Part model, mm, in its own coordinate system. A direction names the side the tool comes from. Round coordinates to 2 decimals unless told otherwise and drop trailing zeros. Write each loop counter-clockwise with the first axis right and the second up, starting at its lowest first coordinate (ties: lowest second). Pieces come first, ordered by that corner, then holes. Notation, with made-up numbers: (73, -0.75) -> (131, -0.75) arc R32 cw to (131, 34.25) -> close; hole circle Ø3 at (-16.75, -36). An arc over 180 degrees is marked (long way). Return JSON: item names as keys, results as strings. Group by question number.
(1) Tool access for faces 4 (the flat face through (-26, 33, -3)), 5 (the flat face through (-49, 32, 198.75)), 6 (the flat face through (2, -19, -198.75)): list every direction of +Z, -Z, +X, -X, +Y, -Y with a clear straight run to the whole face (end or side of a thin tool).
(2) Saw through at C-C (y = 47.5). List the corners of the cut face in (x, z).
(3) Saw through at B-B (x = -12.5). List the corners of the cut face in (y, z).
(4) Mould opens along Z. For faces 1 (the flat face through (2, 0, -3)), 2 (the flat face through (-48, 33, -202.75)), 3 (the cylindrical face through (-43.53, 21.38, 200.78)) say: +Z half, -Z half, draft (parallel to the pull), parting line (faces both ways), or undercut.
(5) Saw through at A-A (z = 122.75). List the corners of the cut face in (x, y), plus the area to 3 significant figures.
(6) Saw through at D-D (z = 3.5). List the corners of the cut face in (x, y).
(7) Drill centre lines: L1, parallel to Z at x = -48, y = 42; L2, parallel to Y at x = 4, z = -93.5; L3, parallel to Y at x = -12, z = 200. Where is each one in solid material? Low to high. Write a range as from..to.
(8) Drop flat-ended pins along their axis: pin 1 Ø1 at (y, z) = (19, -57) entering from +X; pin 2 Ø7.5 at (y, z) = (35, -122.75) entering from -X; pin 3 Ø1.5 at (y, z) = (-9.5, -199) entering from -X; pin 4 Ø3 at (y, z) = (38.5, 108.5) entering from -X. Give the stop position or say it passes through.
from build123d import *

# Parameters (mm, degrees)
SKETCH1_W                      = 60
SKETCH1_H                      = 405.5
BASE_FLANGE1_DEPTH             = 4
EDGE_FLANGE1_STRIP_W           = 18
EDGE_FLANGE1_STRIP_H           = 4
EDGE_FLANGE1_STRIP_CUT_DEPTH   = 405.5
EDGE_FLANGE1_DEPTH             = 405.5
EDGE_FLANGE2_STRIP_W           = 18
EDGE_FLANGE2_STRIP_H           = 4
EDGE_FLANGE2_STRIP_CUT_DEPTH   = 55
EDGE_FLANGE2_STRIP_2_W         = 18
EDGE_FLANGE2_STRIP_2_H         = 4
EDGE_FLANGE2_STRIP_CUT_2_DEPTH = 55
EDGE_FLANGE2_STRIP_3_W         = 18
EDGE_FLANGE2_STRIP_3_H         = 4
EDGE_FLANGE2_STRIP_CUT_3_DEPTH = 55
EDGE_FLANGE2_STRIP_4_W         = 18
EDGE_FLANGE2_STRIP_4_H         = 4
EDGE_FLANGE2_STRIP_CUT_4_DEPTH = 55
EDGE_FLANGE2_DEPTH             = 55
EDGE_FLANGE2_BEND_DEPTH        = 55
EDGE_FLANGE2_BEND_2_DEPTH      = 55
EDGE_FLANGE2_BEND_3_DEPTH      = 55
SKETCH18_R                     = 4.6
EXTRUDE1_DEPTH                 = 416.194231655
SKETCH19_R                     = 4.6
EXTRUDE2_DEPTH                 = 4
SKETCH20_R                     = 4.6
EXTRUDE3_DEPTH                 = 4


# Sheet-metal steps are written as plain solids
with BuildPart() as part:
    # Sketch1 → Base-Flange1 (new body)
    with BuildSketch(Plane(origin=(0, 0, 0), x_dir=(1, 0, 0), z_dir=(0, 1, 0))):
        Rectangle(SKETCH1_W, SKETCH1_H)
    extrude(amount=BASE_FLANGE1_DEPTH)

    # Edge-Flange1 strip (across the edge) → Edge-Flange1 strip cut (cut)
    with BuildSketch(Plane(origin=(-30, 4, -202.75), x_dir=(1, 0, 0), z_dir=(0, 0, 1))):
        with Locations((-4, -2)):
            Rectangle(EDGE_FLANGE1_STRIP_W, EDGE_FLANGE1_STRIP_H)
    extrude(amount=EDGE_FLANGE1_STRIP_CUT_DEPTH, mode=Mode.SUBTRACT)

    # Edge-Flange1 section (across the edge) → Edge-Flange1 (add)
    with BuildSketch(Plane(origin=(-30, 4, -202.75), x_dir=(1, 0, 0), z_dir=(0, 0, 1))):
        with BuildLine():
            Line((0, 1), (0, 56))
            Line((0, 56), (4, 56))
            Line((4, 56), (4, 1))
            ThreePointArc((4, 1), (4.292893219, 0.292893219), (5, 0))
            Line((5, 0), (5, -4))
            ThreePointArc((5, -4), (1.464466094, -2.535533906), (0, 1))
        make_face()
    extrude(amount=EDGE_FLANGE1_DEPTH)

    # Edge-Flange2 strip (across the edge) → Edge-Flange2 strip cut (cut)
    with BuildSketch(Plane(origin=(-30, 5, 202.75), x_dir=(0, 0, -1), z_dir=(0, 1, 0))):
        with Locations((-4, -2)):
            Rectangle(EDGE_FLANGE2_STRIP_W, EDGE_FLANGE2_STRIP_H)
    extrude(amount=EDGE_FLANGE2_STRIP_CUT_DEPTH, mode=Mode.SUBTRACT)

    # Edge-Flange2 strip 2 (across the edge) → Edge-Flange2 strip cut 2 (cut)
    with BuildSketch(Plane(origin=(30, 0, 202.75), x_dir=(0, 0, -1), z_dir=(-1, 0, 0))):
        with Locations((-4, -2)):
            Rectangle(EDGE_FLANGE2_STRIP_2_W, EDGE_FLANGE2_STRIP_2_H)
    extrude(amount=EDGE_FLANGE2_STRIP_CUT_2_DEPTH, mode=Mode.SUBTRACT)

    # Edge-Flange2 strip 3 (across the edge) → Edge-Flange2 strip cut 3 (cut)
    with BuildSketch(Plane(origin=(-30, 60, -202.75), x_dir=(0, 0, 1), z_dir=(0, -1, 0))):
        with Locations((-4, -2)):
            Rectangle(EDGE_FLANGE2_STRIP_3_W, EDGE_FLANGE2_STRIP_3_H)
    extrude(amount=EDGE_FLANGE2_STRIP_CUT_3_DEPTH, mode=Mode.SUBTRACT)

    # Edge-Flange2 strip 4 (across the edge) → Edge-Flange2 strip cut 4 (cut)
    with BuildSketch(Plane(origin=(-25, 0, -202.75), x_dir=(0, 0, 1), z_dir=(1, 0, 0))):
        with Locations((-4, -2)):
            Rectangle(EDGE_FLANGE2_STRIP_4_W, EDGE_FLANGE2_STRIP_4_H)
    extrude(amount=EDGE_FLANGE2_STRIP_CUT_4_DEPTH, mode=Mode.SUBTRACT)

    # Edge-Flange2 section (across the edge) → Edge-Flange2 (add)
    with BuildSketch(Plane(origin=(-30, 5, 202.75), x_dir=(0, 0, -1), z_dir=(0, 1, 0))):
        with BuildLine():
            Line((0, 1), (0, 36))
            Line((0, 36), (4, 36))
            Line((4, 36), (4, 1))
            ThreePointArc((4, 1), (4.292893219, 0.292893219), (5, 0))
            Line((5, 0), (5, -4))
            ThreePointArc((5, -4), (1.464466094, -2.535533906), (0, 1))
        make_face()
    extrude(amount=EDGE_FLANGE2_DEPTH)

    # Edge-Flange2 section 2 (across the edge) → Edge-Flange2 bend (add)
    with BuildSketch(Plane(origin=(30, 0, 202.75), x_dir=(0, 0, -1), z_dir=(-1, 0, 0))):
        with BuildLine():
            Line((0, 1), (0, 36))
            Line((0, 36), (4, 36))
            Line((4, 36), (4, 1))
            ThreePointArc((4, 1), (4.292893219, 0.292893219), (5, 0))
            Line((5, 0), (5, -4))
            ThreePointArc((5, -4), (1.464466094, -2.535533906), (0, 1))
        make_face()
    extrude(amount=EDGE_FLANGE2_BEND_DEPTH)

    # Edge-Flange2 section 3 (across the edge) → Edge-Flange2 bend 2 (add)
    with BuildSketch(Plane(origin=(-30, 60, -202.75), x_dir=(0, 0, 1), z_dir=(0, -1, 0))):
        with BuildLine():
            Line((0, 1), (0, 36))
            Line((0, 36), (4, 36))
            Line((4, 36), (4, 1))
            ThreePointArc((4, 1), (4.292893219, 0.292893219), (5, 0))
            Line((5, 0), (5, -4))
            ThreePointArc((5, -4), (1.464466094, -2.535533906), (0, 1))
        make_face()
    extrude(amount=EDGE_FLANGE2_BEND_2_DEPTH)

    # Edge-Flange2 section 4 (across the edge) → Edge-Flange2 bend 3 (add)
    with BuildSketch(Plane(origin=(-25, 0, -202.75), x_dir=(0, 0, 1), z_dir=(1, 0, 0))):
        with BuildLine():
            Line((0, 1), (0, 36))
            Line((0, 36), (4, 36))
            Line((4, 36), (4, 1))
            ThreePointArc((4, 1), (4.292893219, 0.292893219), (5, 0))
            Line((5, 0), (5, -4))
            ThreePointArc((5, -4), (1.464466094, -2.535533906), (0, 1))
        make_face()
    extrude(amount=EDGE_FLANGE2_BEND_3_DEPTH)

    # Sketch18 → Extrude1 (cut, through all)
    with BuildSketch(Plane.XY.offset(202.75)):
        with Locations((-46, 47.5)):
            Circle(SKETCH18_R)
        with Locations((-46, 17.5)):
            Circle(SKETCH18_R)
        with Locations((-12.5, -16)):
            Circle(SKETCH18_R)
        with Locations((17.5, -16)):
            Circle(SKETCH18_R)
    extrude(amount=-EXTRUDE1_DEPTH, mode=Mode.SUBTRACT)

    # Sketch19 → Extrude2 (cut)
    with BuildSketch(Plane(origin=(-26, 0, 0), x_dir=(0, 0, -1), z_dir=(1, 0, 0))):
        with Locations(Location((-122.75, 35, 0), (0, 0, 90))):
            Circle(SKETCH19_R)
        with Locations(Location((122.75, 35, 0), (0, 0, 90))):
            Circle(SKETCH19_R)
    extrude(amount=-EXTRUDE2_DEPTH, mode=Mode.SUBTRACT)

    # Sketch20 → Extrude3 (cut)
    with BuildSketch(Plane(origin=(0, 4, 0), x_dir=(1, 0, 0), z_dir=(0, 1, 0))):
        with Locations(Location((5, 122.75, 0), (0, 0, 270))):
            Circle(SKETCH20_R)
        with Locations(Location((5, -122.75, 0), (0, 0, 270))):
            Circle(SKETCH20_R)
    extrude(amount=-EXTRUDE3_DEPTH, mode=Mode.SUBTRACT)


solid = part.part
Computed values:
{
 "1": {"face 4": "+Z, -Z, +X, +Y", "face 5": "-X, +Y, -Y", "face 6": "+X, -X, -Y"},
 "2": {"outline": "(-66, -202.75) -> (-50.6, -202.75) -> (-50.6, -198.75) -> (-66, -198.75) -> close; (-66, 198.75) -> (-50.6, 198.75) -> (-50.6, 202.75) -> (-66, 202.75) -> close; (-41.4, -202.75) -> (-31, -202.75) arc R5 ccw to (-26, -197.75) -> (-26, 197.75) arc R5 ccw to (-31, 202.75) -> (-41.4, 202.75) -> (-41.4, 198.75) -> (-31, 198.75) arc R1 cw to (-30, 197.75) -> (-30, -197.75) arc R1 cw to (-31, -198.75) -> (-41.4, -198.75) -> close"},
 "3": {"outline": "(-36, -202.75) -> (-20.6, -202.75) -> (-20.6, -198.75) -> (-36, -198.75) -> close; (-36, 198.75) -> (-20.6, 198.75) -> (-20.6, 202.75) -> (-36, 202.75) -> close; (-11.4, -202.75) -> (-1, -202.75) arc R5 ccw to (4, -197.75) -> (4, 197.75) arc R5 ccw to (-1, 202.75) -> (-11.4, 202.75) -> (-11.4, 198.75) -> (-1, 198.75) arc R1 cw to (0, 197.75) -> (0, -197.75) arc R1 cw to (-1, -198.75) -> (-11.4, -198.75) -> close"},
 "4": {"face 1": "undercut", "face 2": "-Z half", "face 3": "draft"},
 "5": {"outline": "(-30, 5) arc R5 ccw to (-25, 0) -> (0.4, 0) -> (0.4, 4) -> (-25, 4) arc R1 cw to (-26, 5) -> (-26, 30.4) -> (-30, 30.4) -> close; (-30, 39.6) -> (-26, 39.6) -> (-26, 60) -> (-30, 60) -> close; (9.6, 0) -> (30, 0) -> (30, 4) -> (9.6, 4) -> close", "area": "385 mm2"},
 "6": {"outline": "(-30, 5) arc R5 ccw to (-25, 0) -> (30, 0) -> (30, 4) -> (-25, 4) arc R1 cw to (-26, 5) -> (-26, 60) -> (-30, 60) -> close"},
 "7": {"L1": "-202.75..-198.75, 198.75..202.75", "L2": "0..4", "L3": "-36..-20.57, -11.43..3.47"},
 "8": {"pin 1": "x = -26", "pin 2": "through", "pin 3": "x = -25", "pin 4": "x = -30"}
}
